Input: part model. Units: mm. Frame: model coordinates. Face numbers are marked on the shaded views. Give positions to 0.01 mm unless a question says otherwise; leave off trailing zeros. Loops run counter-clockwise (first coordinate to the right, second up) from the corner with the lowest first, then second, coordinate; pieces in that order, holes last. Notation, with made-up numbers: M -11.5,3 L 22.5,3 A15 cw 22.5,18 Z; hole C 20,85 d7. An arc over 180 degrees is marked long. Use CSV: the item, a comma, the result in double quotes. Start each with the question number.
Q1. Pull-direction query (Y, two-part tool) for the marked faces 1, 2 and 3; classes: released by +Y, released by -Y, zero draft, split by the parting line, or undercut.
Q2. Section B-B, the plane x = -8.5. Output: boundary loops of the cut face in (y, z), plus the area to 3 significant figures.
Q3. Material intervals for line 1 along Y through (x, z) = (0, 8.25); line 2 along X through (y, z) = (-0.5, 5); line 3 along Y through (x, z) = (8.5, 6.5), sorted ascending.
Q4. Section D-D, the plane z = 1.25. Output: boundary loops of the cut face in (x, y).
Q5. Pin query (flat end, axial travel): pin 1 (2.5 mm diameter, centred on x = 0, y = -8.5, fed in from +Z); pin 2 (5 mm diameter, centred on y = -6.5, z = 7.5, fed in from -X); pin 3 (1 mm diameter, centred on x = -9, z = 5, fed in from -Y); pin 4 (6 mm diameter, centred on y = 13, z = 7, fed in from -X). Return the tip coordinate at first contact, or that it passes through.
Q6. Section A-A, the plane y = 0. Output: boundary loops of the cut face in (x, z), plus the area to 3 significant figures.
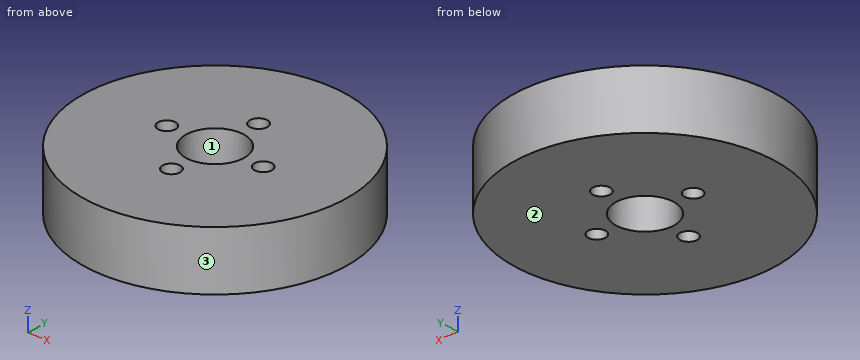
from build123d import *

# Parameters (mm, degrees)
ESQUISSE1_R        = 22.5
ESQUISSE1_R_2      = 5
BOSS_EXTRU_1_DEPTH = 10
D_GAGEMENT_M21_D   = 3


with BuildPart() as part:
    # Esquisse1 → Boss.-Extru.1 (new body)
    with BuildSketch(Plane.XY):
        Circle(ESQUISSE1_R)
        Circle(ESQUISSE1_R_2, mode=Mode.SUBTRACT)
    extrude(amount=BOSS_EXTRU_1_DEPTH)

    # Dégagement M21 (through all)
    with Locations(Plane.XY.offset(10)):
        with Locations((0, 8.5), (8.5, 0), (0, -8.5), (-8.5, 0), (0, 0)):
            Hole(D_GAGEMENT_M21_D / 2)


solid = part.part
A:
1,face 1,"undercut"
1,face 2,"zero draft"
1,face 3,"split by the parting line"
2,outline,"M -20.83,0 L -1.5,0 L -1.5,10 L -20.83,10 Z; M 1.5,0 L 20.83,0 L 20.83,10 L 1.5,10 Z"
2,area,"387 mm^2"
3,line 1,"-22.5 to -10, -7 to -5, 5 to 7, 10 to 22.5"
3,line 2,"-22.49 to -9.91, -7.09 to -4.97, 4.97 to 7.09, 9.91 to 22.49"
3,line 3,"-20.83 to -1.5, 1.5 to 20.83"
4,outline,"C 0,0 d45; hole C -8.5,0 d3; hole C 0,0 d10; hole C 0,-8.5 d3; hole C 0,8.5 d3; hole C 8.5,0 d3"
5,pin 1,"through"
5,pin 2,"x = -22.14"
5,pin 3,"y = -20.83"
5,pin 4,"x = -20.16"
6,outline,"M -22.5,0 L -10,0 L -10,10 L -22.5,10 Z; M -7,0 L -5,0 L -5,10 L -7,10 Z; M 5,0 L 7,0 L 7,10 L 5,10 Z; M 10,0 L 22.5,0 L 22.5,10 L 10,10 Z"
6,area,"290 mm^2"
